```python
from build123d import *

# Parameters (mm, degrees)
SKETCH1_W                      = 290
SKETCH1_H                      = 40
BASE_FLANGE1_DEPTH             = 3
EDGE_FLANGE1_STRIP_W           = 13.4732
EDGE_FLANGE1_STRIP_H           = 3
EDGE_FLANGE1_STRIP_CUT_DEPTH   = 40
EDGE_FLANGE1_DEPTH             = 40
EDGE_FLANGE2_STRIP_W           = 13.4732
EDGE_FLANGE2_STRIP_H           = 3
EDGE_FLANGE2_STRIP_CUT_DEPTH   = 40
EDGE_FLANGE2_DEPTH             = 40
F_8_0MM_DOWEL_HOLE1_AT_2_COUNT = 2
F_8_0MM_DOWEL_HOLE1_AT_2_PITCH = 162.5268


# Sheet-metal steps are written as plain solids
with BuildPart() as part:
    # Sketch1 → Base-Flange1 (new body)
    with BuildSketch(Plane.XY):
        with Locations((145, 20)):
            Rectangle(SKETCH1_W, SKETCH1_H)
    extrude(amount=-BASE_FLANGE1_DEPTH)

    # Edge-Flange1 strip (across the edge) → Edge-Flange1 strip cut (cut)
    with BuildSketch(Plane.XZ.offset(-40)):
        with Locations((-3, -1.5)):
            Rectangle(EDGE_FLANGE1_STRIP_W, EDGE_FLANGE1_STRIP_H)
    extrude(amount=EDGE_FLANGE1_STRIP_CUT_DEPTH, mode=Mode.SUBTRACT)

    # Edge-Flange1 section (across the edge) → Edge-Flange1 (add)
    with BuildSketch(Plane.XZ.offset(-40)):
        with BuildLine():
            Line((0, 0.7366), (0, 17))
            Line((0, 17), (3, 17))
            Line((3, 17), (3, 0.7366))
            ThreePointArc((3, 0.7366), (3.215745145, 0.215745145), (3.7366, 0))
            Line((3.7366, 0), (3.7366, -3))
            ThreePointArc((3.7366, -3), (1.094424801, -1.905575199), (0, 0.7366))
        make_face()
    extrude(amount=EDGE_FLANGE1_DEPTH)

    # Edge-Flange2 strip (across the edge) → Edge-Flange2 strip cut (cut)
    with BuildSketch(Plane(origin=(290, 0, 0), x_dir=(-1, 0, 0), z_dir=(0, 1, 0))):
        with Locations((-3, -1.5)):
            Rectangle(EDGE_FLANGE2_STRIP_W, EDGE_FLANGE2_STRIP_H)
    extrude(amount=EDGE_FLANGE2_STRIP_CUT_DEPTH, mode=Mode.SUBTRACT)

    # Edge-Flange2 section (across the edge) → Edge-Flange2 (add)
    with BuildSketch(Plane(origin=(290, 0, 0), x_dir=(-1, 0, 0), z_dir=(0, 1, 0))):
        with BuildLine():
            Line((0, 0.7366), (0, 17))
            Line((0, 17), (3, 17))
            Line((3, 17), (3, 0.7366))
            ThreePointArc((3, 0.7366), (3.215745145, 0.215745145), (3.7366, 0))
            Line((3.7366, 0), (3.7366, -3))
            ThreePointArc((3.7366, -3), (1.094424801, -1.905575199), (0, 0.7366))
        make_face()
    extrude(amount=EDGE_FLANGE2_DEPTH)

    # Sketch13 → Ø8.0mm Dowel Hole1 (revolve, cut)
    with BuildSketch(Plane(origin=(226.2634, 20, 0), x_dir=(0, -1, 0), z_dir=(1, 0, 0))):
        Polygon((0, 0), (0, 3), (4, 3), (4, 0.025), (4.025, 0), align=None)
    f_8_0mm_dowel_hole1 = revolve(axis=Axis((226.2634, 20, 6.35), (0, 0, -1)), mode=Mode.SUBTRACT)

    # Ø8.0mm Dowel Hole1 at 2: Ø8.0mm Dowel Hole1 ×2
    with Locations(*[(-i * F_8_0MM_DOWEL_HOLE1_AT_2_PITCH, 0, 0) for i in range(1, F_8_0MM_DOWEL_HOLE1_AT_2_COUNT)]):
        add(f_8_0mm_dowel_hole1, mode=Mode.SUBTRACT)


solid = part.part
```
Read the model definition and answer for the solid it produces. Units are mm, in the model's axes. A direction names the side the tool comes from. Give positions to 0.01 mm unless a question says otherwise; leave off trailing zeros. Order: outer loops, then holes, each group sorted by start corner. A loop starts at its lowest first (then second) coordinate and runs counter-clockwise, first axis right, second up.
(1) Find section B-B (y = 20). Give the vertices of the cut face in (x, z) (3 decimals), plus the area to 3 significant figures.
(2) Straight lines are drawn through the part: L1, parallel to X at y = 9.5, z = 8.5; L2, parallel to X at y = 20, z = -1.5; L3, parallel to X at y = 20, z = -0.7. For each, find the intervals that lie inside material, in ascending order.
(3) Find section C-C (y = 31.5). Give the vertices of the cut face in (x, z), plus the area to 3 significant figures.
(4) Given pin 1 (6.5 mm diameter, centred on x = 226.26, y = 20, fed in from +Z); pin 2 (9 mm diameter, centred on x = 63.74, y = 20, fed in from +Z), each flat-ended and moving along its own axis, determine where each tip first touches the part or whether it passes through.
(5) Find section D-D (x = 96). Give the vertices of the cut face in (y, z), plus the area to 3 significant figures.
(6) For a pull along X with two mould halves and no side action, classify faces 3 (the flat face through (144, 0, -1)), 4 (the flat face through (287, 20, 9)), 5 (the flat face through (0, 20, 9)) as released by +X, released by -X, zero draft, split by the parting line, or undercut.
(7) Find section A-A (z = 9.25). Give the vertices of the cut face in (x, y).
(8) For faces 1 (the flat face through (3, 20, 9)), 2 (the flat face through (290, 20, 9)), determine the directions among +Z, -Z, +X, -X, +Y, -Y from which every point of the face is accessible in a straight line to the end or side of a thin tool.
Result sheet:
1. outline: (0, 0.737) arc R3.737 ccw to (3.737, -3) - (59.737, -3) - (59.737, -0.025) - (59.712, 0) - (3.737, 0) arc R0.737 cw to (3, 0.737) - (3, 17) - (0, 17) - close; (67.737, -3) - (222.263, -3) - (222.263, -0.025) - (222.238, 0) - (67.762, 0) - (67.737, -0.025) - close; (230.263, -3) - (286.263, -3) arc R3.737 ccw to (290, 0.737) - (290, 17) - (287, 17) - (287, 0.737) arc R0.737 cw to (286.263, 0) - (230.288, 0) - (230.263, -0.025) - close
1. area: 918 mm2
2. L1: x = 0 to 3, 287 to 290
2. L2: x = 0.74 to 59.74, 67.74 to 222.26, 230.26 to 289.26
2. L3: x = 0.29 to 59.74, 67.74 to 222.26, 230.26 to 289.71
3. outline: (0, 0.74) arc R3.74 ccw to (3.74, -3) - (286.26, -3) arc R3.74 ccw to (290, 0.74) - (290, 17) - (287, 17) - (287, 0.74) arc R0.74 cw to (286.26, 0) - (3.74, 0) arc R0.74 cw to (3, 0.74) - (3, 17) - (0, 17) - close
3. area: 966 mm2
4. pin 1: passes through
4. pin 2: stops at z = 0
5. outline: (0, -3) - (40, -3) - (40, 0) - (0, 0) - close
5. area: 120 mm2
6. face 3: zero draft
6. face 4: undercut
6. face 5: released by -X
7. outline: (0, 0) - (3, 0) - (3, 40) - (0, 40) - close; (287, 0) - (290, 0) - (290, 40) - (287, 40) - close
8. face 1: +Z, +Y, -Y
8. face 2: +Z, -Z, +X, +Y, -Y
